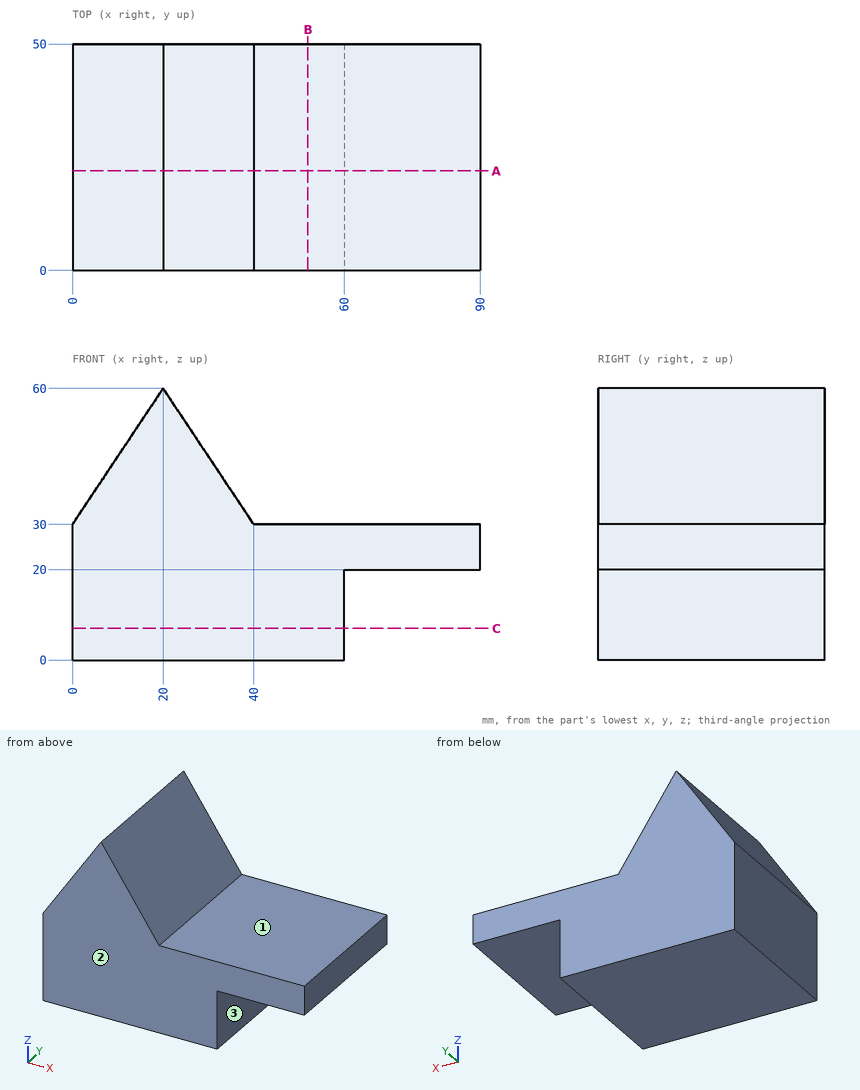
Drawing for the job (mm, zero at the part's lowest x, y, z). A direction names the side the tool comes from. Round coordinates to 2 decimals unless told otherwise and drop trailing zeros. Order: outer loops, then holes, each group sorted by start corner. A loop starts at its lowest first (then second) coordinate and runs counter-clockwise, first axis right, second up. Notation, with made-up numbers: (-10.75, 20) -> (25.25, 20) arc R26 cw to (25.25, 59) -> close; hole circle Ø4 at (16, -32.75). An arc over 180 degrees is marked (long way). Put each result on its own line as item: value.
Q1. Band-saw the part on A-A (y = 22). Give the cut face in (x, z).
From the geometry:
outline: (0, 0) -> (60, 0) -> (60, 20) -> (90, 20) -> (90, 30) -> (40, 30) -> (20, 60) -> (0, 30) -> close
Q2. Tool access for the marked faces 1, 2 and 3: list every direction of +Z, -Z, +X, -X, +Y, -Y with a clear straight run to the whole face (end or side of a thin tool).
From the geometry:
face 1: +Z, +X, +Y, -Y
face 2: +Z, -Z, +X, -X, -Y
face 3: -Z, +X, +Y, -Y
Q3. Wall check: line 1 (Z direction, x = 50.5, y = 42); line 2 (X direction, y = 43.5, z = 9); line 3 (Z direction, x = 63, y = 18.5). Give the ranges that are in metal, low to high. Write a range as [from, to].
From the geometry:
line 1: z = [0, 30]
line 2: x = [0, 60]
line 3: z = [20, 30]
Q4. Pin check, flat tips, straight feed: pin 1 Ø8 at (x, z) = (11, 32) entering from -Y; pin 2 Ø2 at (x, y) = (10, 8) entering from +Z; pin 3 Ø10 at (y, z) = (35.5, 13.5) entering from +X; pin 4 Ø25 at (x, y) = (74.5, 14) entering from +Z. Stop position of each tip, or through.
From the geometry:
pin 1: stops at y = 0
pin 2: stops at z = 46.5
pin 3: stops at x = 60
pin 4: stops at z = 30
Q5. Band-saw the part on B-B (x = 52). Give the cut face in (y, z).
From the geometry:
outline: (0, 0) -> (50, 0) -> (50, 30) -> (0, 30) -> close
Q6. Band-saw the part on C-C (z = 7). Give the cut face in (x, y), and give its area (3 significant figures).
From the geometry:
outline: (0, 0) -> (60, 0) -> (60, 50) -> (0, 50) -> close
area: 3,000 mm2
